Work out the finished part from the listing and answer in its coordinate system (mm). Face numbers are marked on the shaded views. Round coordinates to 2 decimals unless told otherwise and drop trailing zeros. Loops run counter-clockwise (first coordinate to the right, second up) from the corner with the lowest first, then second, coordinate; pieces in that order, holes last. Notation, with made-up numbers: (72, -16.75) -> (88, -16.75) arc R15 cw to (88, 10.25) -> close; hole circle Ø8 at (-32.75, 76.25). An arc over 180 degrees is marked (long way). Use CSV: the item, a comma, the result in double quotes. Start each with the question number.
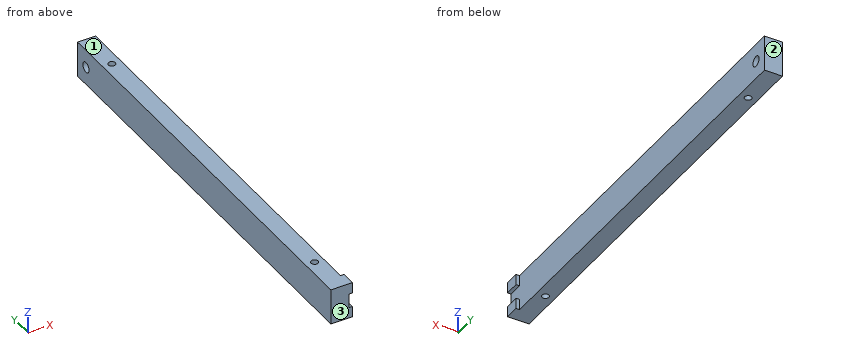
from build123d import *

# Parameters (mm, degrees)
BOSS_EXTRUDE1_DEPTH = 190.5
SKETCH2_W           = 1.5875
SKETCH2_H           = 15.875
CUT_EXTRUDE1_DEPTH  = 184.15
SKETCH3_R           = 1.524
CUT_EXTRUDE2_DEPTH  = 192.397469288
SKETCH4_R           = 2.286
CUT_EXTRUDE3_DEPTH  = 192.397469288


with BuildPart() as part:
    # Sketch1 → Boss-Extrude1 (new body)
    with BuildSketch(Plane(origin=(0, 0, 0), x_dir=(1, 0, 0), z_dir=(0, 1, 0))):
        Polygon((0, 0), (0, -15.875), (9.525, -15.875), (9.525, -11.1125), (7.9375, -11.1125), (7.9375, -4.7625), (9.525, -4.7625), (9.525, 0), align=None)
    extrude(amount=BOSS_EXTRUDE1_DEPTH)

    # Sketch2 → Cut-Extrude1 (cut)
    with BuildSketch(Plane(origin=(0, 190.5, 0), x_dir=(1, 0, 0), z_dir=(0, 1, 0))):
        with Locations((8.73125, -7.9375)):
            Rectangle(SKETCH2_W, SKETCH2_H)
    extrude(amount=-CUT_EXTRUDE1_DEPTH, mode=Mode.SUBTRACT)

    # Sketch3 → Cut-Extrude2 (cut, through all)
    with BuildSketch(Plane.XY.offset(15.875)):
        with Locations((3.96875, 19.05)):
            Circle(SKETCH3_R)
        with Locations((3.96875, 171.45)):
            Circle(SKETCH3_R)
    extrude(amount=-CUT_EXTRUDE2_DEPTH, mode=Mode.SUBTRACT)

    # Sketch4 → Cut-Extrude3 (cut, through all)
    with BuildSketch(Plane.ZY):
        with Locations((7.9375, 184.15)):
            Circle(SKETCH4_R)
    extrude(amount=-CUT_EXTRUDE3_DEPTH, mode=Mode.SUBTRACT)


solid = part.part
Q1. Section B-B, the plane x = 4 is taken. Give the number of separate pieces and of enclosed holes in the cut face, and give its area (3 significant figures).
Q2. Section C-C, the plane y = 69.5 is taken. Write down the section's boundary in (x, z) (1 decimal).
Q3. Straight lines are drawn through the part: line 1 (Y direction, x = 4, z = 15); line 2 (Z direction, x = 4.25, y = 184.15) (1 decimal); line 3 (Y direction, x = 6, z = 8). For each, find the intervals that lie inside material, in ascending order. Write a range as from..to.
Q4. Each of these flat-tipped pins is pushed along its axis until it touches: pin 1 (1 mm diameter, centred on y = 162, z = 13, fed in from +X); pin 2 (0.5 mm diameter, centred on x = 8.5, z = 2.5, fed in from +Y); pin 3 (1 mm diameter, centred on y = 116.5, z = 6.5, fed in from -X); pin 4 (1.8 mm diameter, centred on x = 3.97, y = 19.05, fed in from -Z). Where does it stop, or does it pass through?
Q5. Section A-A, the plane y = 184.15 is taken. Write down the section's boundary in (x, z) (1 decimal), and give its area (3 significant figures).
Q6. For a pull along Y with two mould halves and no side action, classify the marked faces 1, 2 and 3 as pulls with the +Y half, pulls with the -Y half, needs draft (parallel to the pull), parting line crosses it, or undercut.
Report:
1,separate pieces,"3"
1,enclosed holes,"1"
1,area,"2,910 mm²"
2,outline,"(0, 0) -> (7.9, 0) -> (7.9, 15.9) -> (0, 15.9) -> close"
3,line 1,"y = 0..17.53, 20.57..169.93, 172.97..190.5"
3,line 2,"z = 0..5.7, 10.2..15.9"
3,line 3,"y = 0..181.86, 186.44..190.5"
4,pin 1,"stops at x = 7.94"
4,pin 2,"stops at y = 6.35"
4,pin 3,"stops at x = 0"
4,pin 4,"passes through"
5,outline,"(0, 0) -> (7.9, 0) -> (7.9, 5.7) -> (0, 5.7) -> close; (0, 10.2) -> (7.9, 10.2) -> (7.9, 15.9) -> (0, 15.9) -> close"
5,area,"89.7 mm²"
6,face 1,"needs draft"
6,face 2,"pulls with the +Y half"
6,face 3,"pulls with the -Y half"
